from build123d import *

# Parameters (mm, degrees)
F1_DEPTH = 2.54


with BuildPart() as f1:
    # F0 (on Top) → F1 (new body)
    with BuildSketch(Plane.XY):
        with BuildLine():
            Line((0, 10.16), (0, 0))
            Line((0, 0), (29.1318279277, 0))
            ThreePointArc((29.1318279277, 0), (26.035, 5.08), (29.1318279277, 10.16))
            Line((29.1318279277, 10.16), (0, 10.16))
        make_face()
        with BuildLine():
            ThreePointArc((29.1318279277, 10.16), (26.035, 5.08), (29.1318279277, 0))
            Line((29.1318279277, 0), (31.75, 0))
            Line((31.75, 0), (31.75, 0.889))
            ThreePointArc((31.75, 0.889), (27.559, 5.08), (31.75, 9.271))
            Line((31.75, 9.271), (31.75, 10.16))
            Line((31.75, 10.16), (29.1318279277, 10.16))
        make_face()
        with BuildLine():
            Line((31.75, 0), (29.1318279277, 0))
            ThreePointArc((29.1318279277, 0), (34.7247581084, 0.2002418916), (37.465, 5.08))
            ThreePointArc((37.465, 5.08), (34.7247581084, 9.9597581084), (29.1318279277, 10.16))
            Line((29.1318279277, 10.16), (31.75, 10.16))
            Line((31.75, 10.16), (31.75, 9.271))
            ThreePointArc((31.75, 9.271), (34.71348452, 8.04348452), (35.941, 5.08))
            ThreePointArc((35.941, 5.08), (34.71348452, 2.11651548), (31.75, 0.889))
            Line((31.75, 0.889), (31.75, 0))
        make_face()
    extrude(amount=F1_DEPTH)


solid = f1.part
Work out the finished part from the listing and answer in its coordinate system (mm). A direction names the side the tool comes from. Coordinates: 2 decimals unless noted, no trailing zeros. Loops run counter-clockwise (first coordinate to the right, second up) from the corner with the lowest first, then second, coordinate; pieces in that order, holes last. Notation, with made-up numbers: (3.25, 36) -> (28.25, 36) arc R28 ccw to (28.25, 69) -> close; hole circle Ø10 at (75.5, -14). An arc over 180 degrees is marked (long way). Write each question's results on one line, items separated by ' | '. Start each with the question number.
1) Find section C-C on x = 7.5. Determine the outline of the cut face in (y, z), then the cut area to 3 significant figures.
2) Consider line 1 along Y through (x, z) = (12.5, 2); line 2 along X through (y, z) = (1.5, 1.9); line 3 along Y through (x, z) = (34.5, 2.1). Determine where each line is inside the solid, lowest interval first.
3) Find section A-A on z = 1.7. Determine the outline of the cut face in (x, y) (3 decimals).
4) Find section B-B on y = 3.75. Determine the outline of the cut face in (x, z).
5) Flat-ended cylindrical pins translate along their axes: P1, Ø0.8, axis at x = 8, z = 0.5, coming from the +Y side; P2, Ø1.3, axis at x = 7.5, z = 1, coming from the -Y side; P3, Ø1.5, axis at x = 33.5, z = 2, coming from the -Y side; P4, Ø1.5, axis at x = 29, y = 5.5, coming from the -Z side. Find the tip coordinate at first contact, or state that the pin passes through.
6) For faces 1 (the flat face through (14, 0, 1)), 2 (the flat face through (0, 5, 1)), 3 (the flat face through (15, 10.16, 1)), determine the directions among +Z, -Z, +X, -X, +Y, -Y from which every point of the face is accessible in a straight line to the end or side of a thin tool.
Response values:
1) outline: (0, 0) -> (10.16, 0) -> (10.16, 2.54) -> (0, 2.54) -> close | area: 25.8 mm^2
2) line 1: y = 0 to 10.16 | line 2: x = 0 to 29.57, 33.93 to 36.2 | line 3: y = 0.07 to 1.92, 8.24 to 10.09
3) outline: (0, 0) -> (29.132, 0) arc R5.715 ccw (long way) to (29.132, 10.16) -> (0, 10.16) -> close; hole circle Ø8.382 at (31.75, 5.08)
4) outline: (0, 0) -> (27.78, 0) -> (27.78, 2.54) -> (0, 2.54) -> close; (35.72, 0) -> (37.31, 0) -> (37.31, 2.54) -> (35.72, 2.54) -> close
5) P1: stops at y = 10.16 | P2: stops at y = 0 | P3: stops at y = -0.55 | P4: passes through
6) face 1: +Z, -Z, -X, -Y | face 2: +Z, -Z, -X, +Y, -Y | face 3: +Z, -Z, -X, +Y
